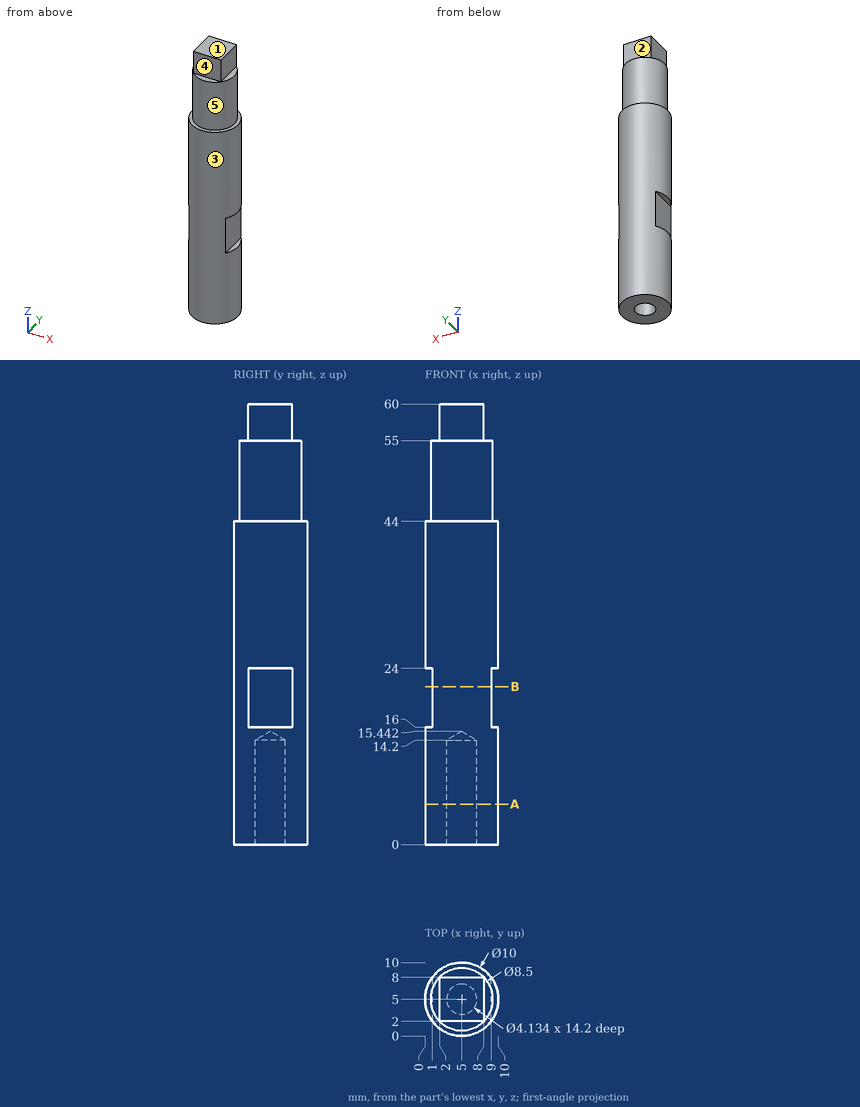
The figure shows three views and two pictorial views of one solid part (mm, origin at its lowest corner). Answer the questions. A direction names the side the tool comes from. Round coordinates to 2 decimals unless told otherwise and drop trailing zeros. Order: outer loops, then holes, each group sorted by start corner. A loop starts at its lowest first (then second) coordinate and runs counter-clockwise, first axis right, second up. Notation, with made-up numbers: M -5,-0.5 L 53,-0.5 A33 cw 53,28.5 Z; hole C -4.5,9.5 d8. An arc over 180 degrees is marked long. Put each result on its own line as item: value. Start each with the question number.
Q1. A tool of negligible diameter and unlimited length cuts with its end or side. For the marked faces 1, 2, 3, 4 and 5, from which of +Z, -Z, +X, -X, +Y, -Y can it reach the whole face along a straight path? Write none if from no direction.
Q2. Flat-ended cylindrical pins translate along their axes: pin 1 (3 mm diameter, centred on x = 4.5, z = 17, fed in from -Y); pin 2 (2.5 mm diameter, centred on y = 4.5, z = 58, fed in from -X); pin 3 (1.5 mm diameter, centred on x = 2.5, z = 42, fed in from +Y); pin 4 (5.5 mm diameter, centred on x = 6.5, z = 58, fed in from +Y). Find the tip coordinate at first contact, or state that the pin passes through.
Q3. Straight lines are drawn through the part: L1, parallel to Y at x = 5, z = 5; L2, parallel to Y at x = 1, z = 39. For each, find the intervals that lie inside material, in ascending order. Write a range as [from, to].
Q4. Section B-B, the plane z = 21.5 is taken. Write down the section's boundary in (x, y), and give its area (3 significant figures).
Q5. Section A-A, the plane z = 5.5 is taken. Write down the section's boundary in (x, y).
Findings below:
1. face 1: +Z, +X, -X, +Y, -Y
1. face 2: +Z, +X, -X, +Y
1. face 3: +Z, -Z
1. face 4: +Z, +X, -X, -Y
1. face 5: +Z
2. pin 1: stops at y = 0
2. pin 2: stops at x = 2
2. pin 3: stops at y = 9.68
2. pin 4: stops at y = 8
3. L1: y = [0, 2.93], [7.07, 10]
3. L2: y = [2, 8]
4. outline: M 1,2 A5 ccw 9,2 L 9,8 A5 ccw 1,8 Z
4. area: 70.4 mm^2
5. outline: C 5,5 d10; hole C 5,5 d4.13
